```python
from build123d import *

# Parameters (mm, degrees)
F0_W     = 48.799998641
F0_H     = 16.799998641
F0_W_2   = 44.799998641
F0_H_2   = 12.799998641
F0_W_3   = 44
F0_H_3   = 12
F0_W_4   = 40
F0_H_4   = 8
F1_DEPTH = 45
F2_DEPTH = 42
F3_DEPTH = 10
F4_R     = 2
F5_R     = 2
F6_R     = 2
F8_DEPTH = 25.2
F9_R     = 8.19999


# Not quite as in the source:
# - a fillet or chamfer is up to 0.001 mm smaller than in the source, because OpenCascade refuses the exact size


with BuildPart() as f1:
    # F0 (on Top) → F1 (new body)
    with BuildSketch(Plane.XY):
        with Locations((-3.2957775742, 1.1005828176)):
            Rectangle(F0_W, F0_H)
        with Locations((-3.2957775742, 1.1005828176)):
            Rectangle(F0_W_2, F0_H_2, mode=Mode.SUBTRACT)
        with Locations((-3.2957775742, 1.1005828176)):
            Rectangle(F0_W_2, F0_H_2)
        with Locations((-3.2957775742, 1.1005828176)):
            Rectangle(F0_W_3, F0_H_3, mode=Mode.SUBTRACT)
        with Locations((-3.2957775742, 1.1005828176)):
            Rectangle(F0_W_3, F0_H_3)
        with Locations((-3.2957775742, 1.1005828176)):
            Rectangle(F0_W_4, F0_H_4, mode=Mode.SUBTRACT)
        with Locations((-3.2957775742, 1.1005828176)):
            Rectangle(F0_W_4, F0_H_4)
    extrude(amount=F1_DEPTH)

    # F0 (on Top) → F2 (cut)
    with BuildSketch(Plane.XY):
        with Locations((-3.2957775742, 1.1005828176)):
            Rectangle(F0_W_4, F0_H_4)
    extrude(amount=F2_DEPTH, mode=Mode.SUBTRACT)

    # F0 (on Top) → F3 (join)
    with BuildSketch(Plane.XY):
        with Locations((-3.2957775742, 1.1005828176)):
            Rectangle(F0_W_3, F0_H_3)
        with Locations((-3.2957775742, 1.1005828176)):
            Rectangle(F0_W_4, F0_H_4, mode=Mode.SUBTRACT)
    extrude(amount=-F3_DEPTH)

    # F4
    f4_edges = [f1.edges().sort_by_distance(p)[0] for p in [
        (-27.695777, -7.299417, 22.5),
        (-27.695777, 9.500582, 22.5),
        (21.104222, -7.299417, 22.5),
        (21.104222, 9.500582, 22.5),
    ]]
    fillet(f4_edges, radius=F4_R)

    # F5
    f5_edges = [f1.edges().sort_by_distance(p)[0] for p in [
        (-23.295778, 5.100583, 16),
        (-23.295778, -2.899417, 16),
        (16.704222, 5.100583, 16),
        (16.704222, -2.899417, 16),
    ]]
    fillet(f5_edges, radius=F5_R)

    # F6
    f6_edges = [f1.edges().sort_by_distance(p)[0] for p in [
        (18.704222, -4.899417, -5),
        (18.704222, 7.100583, -5),
        (-25.295778, -4.899417, -5),
        (-25.295778, 7.100583, -5),
    ]]
    fillet(f6_edges, radius=F6_R)

    # F7 (on face) → F8 (cut)
    with BuildSketch(Plane(origin=(0, 0, 0), x_dir=(1, 0, 0), z_dir=(0, 0, -1))):
        Polygon((4.9042224258, 7.2994165029), (-3.2957775742, 7.2994165029), (-11.4957775742, 7.2994165029), (-11.4957775742, 5.1994165029), (4.9042224258, 5.1994165029), align=None)
        Polygon((-3.2957775742, -9.5005821381), (4.9042224258, -9.5005821381), (4.9042224258, -7.4005821381), (-11.4957775742, -7.4005821381), (-11.4957775742, -9.5005821381), align=None)
    extrude(amount=-F8_DEPTH, mode=Mode.SUBTRACT)

    # F9 (radius 8.2 in the source; OpenCascade refuses exactly that, so slightly less here)
    f9_edges = [f1.edges().sort_by_distance(p)[0] for p in [
        (-11.495778, -6.249417, 25.2),
        (4.904222, -6.249417, 25.2),
        (4.904222, 8.450582, 25.2),
        (-11.495778, 8.450582, 25.2),
    ]]
    fillet(f9_edges, radius=F9_R)


solid = f1.part
```
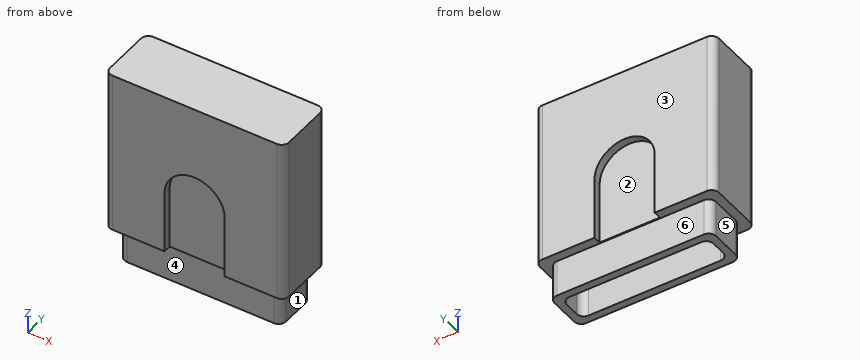
Check sheet for the modelled part. Datum: model origin and axes. Units: mm. Face numbers are marked on the shaded views. A direction names the side the tool comes from. Round coordinates to 2 decimals unless told otherwise and drop trailing zeros. Loops run counter-clockwise (first coordinate to the right, second up) from the corner with the lowest first, then second, coordinate; pieces in that order, holes last. Notation, with made-up numbers: M 32.5,15.25 L 46.5,15.25 A20 ccw 46.5,36.25 Z; hole C -19,-12 d6. An arc over 180 degrees is marked long. Answer as a JSON object with one key per item and string values.
1. Gauge pin test, flat ends, axial feed: P1, Ø3, axis at x = -7, z = -7, coming from the +Y side; P2, Ø4, axis at x = -9.5, y = 1.5, coming from the -Z side; P3, Ø8, axis at x = 5, z = -5.5, coming from the -Y side. Record the tip position at first contact, or that the pin passes through.
Reply:
{"P1": "stops at y = 7.1", "P2": "stops at z = 42", "P3": "stops at y = -4.9"}
2. Mould release check, pull along X, two halves, no side actions. Record for the marked faces 1, 2 and 3: pulls with the +X half, pulls with the -X half, needs draft (parallel to the pull), parting line crosses it, or undercut.
Reply:
{"face 1": "pulls with the +X half", "face 2": "undercut", "face 3": "needs draft"}
3. Section check D-D (z = -1.5). Record the boundary of the cut face in (x, y), plus the area to 3 significant figures.
Reply:
{"outline": "M -25.3,-2.9 A2 ccw -23.3,-4.9 L 16.7,-4.9 A2 ccw 18.7,-2.9 L 18.7,5.1 A2 ccw 16.7,7.1 L -23.3,7.1 A2 ccw -25.3,5.1 Z; hole M -23.3,-0.9 A2 ccw -21.3,-2.9 L 14.7,-2.9 A2 ccw 16.7,-0.9 L 16.7,3.1 A2 ccw 14.7,5.1 L -21.3,5.1 A2 ccw -23.3,3.1 Z", "area": "208 mm²"}
4. Section check B-B (x = 12). Record the boundary of the cut face in (y, z).
Reply:
{"outline": "M -7.3,0 L -4.9,0 L -4.9,-10 L -2.9,-10 L -2.9,42 L 5.1,42 L 5.1,-10 L 7.1,-10 L 7.1,0 L 9.5,0 L 9.5,45 L -7.3,45 Z"}
5. Section check A-A (z = 8). Record the boundary of the cut face in (x, y).
Reply:
{"outline": "M -27.7,-5.3 A2 ccw -25.7,-7.3 L -11.5,-7.3 L -11.5,-5.2 L 4.9,-5.2 L 4.9,-7.3 L 19.1,-7.3 A2 ccw 21.1,-5.3 L 21.1,7.5 A2 ccw 19.1,9.5 L 4.9,9.5 L 4.9,7.4 L -11.5,7.4 L -11.5,9.5 L -25.7,9.5 A2 ccw -27.7,7.5 Z; hole M -23.3,-0.9 A2 ccw -21.3,-2.9 L 14.7,-2.9 A2 ccw 16.7,-0.9 L 16.7,3.1 A2 ccw 14.7,5.1 L -21.3,5.1 A2 ccw -23.3,3.1 Z"}
6. Scan lines: line 1 (Y direction, x = -16.5, z = 26.5); line 2 (X direction, y = 2.75, z = 11); line 3 (Y direction, x = 0.5, z = -6.5). Record each from-to range of solid material in increasing order.
Reply:
{"line 1": "y = -7.3 to -2.9, 5.1 to 9.5", "line 2": "x = -27.7 to -23.3, 16.7 to 21.1", "line 3": "y = -4.9 to -2.9, 5.1 to 7.1"}
7. Section check C-C (y = 1.5). Record the boundary of the cut face in (x, z), plus the area to 3 significant figures.
Reply:
{"outline": "M -27.7,0 L -25.3,0 L -25.3,-10 L -23.3,-10 L -23.3,42 L 16.7,42 L 16.7,-10 L 18.7,-10 L 18.7,0 L 21.1,0 L 21.1,45 L -27.7,45 Z", "area": "556 mm²"}
8. Access from +Z, -Z, +X, -X, +Y, -Y to the whole of each face (thin tool, end or side, straight path). Record for the marked faces 4, 5 and 6.
Reply:
{"face 4": "-Z, +X, -X, -Y", "face 5": "-Z, -X, +Y, -Y", "face 6": "-Z, +X, -X, +Y"}
